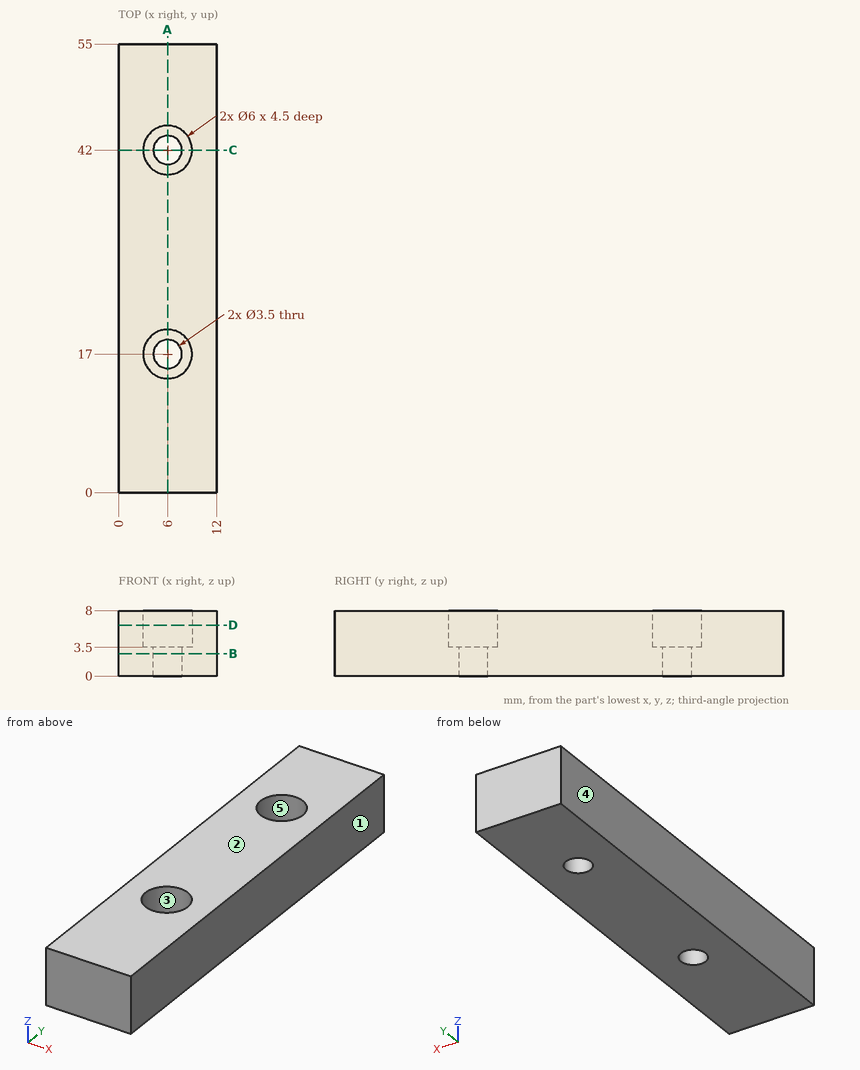
The figure shows three views and two pictorial views of one solid part (mm, origin at its lowest corner). Answer the questions. A direction names the side the tool comes from. Round coordinates to 2 decimals unless told otherwise and drop trailing zeros. Order: outer loops, then holes, each group sorted by start corner. A loop starts at its lowest first (then second) coordinate and runs counter-clockwise, first axis right, second up.
Q1. A tool of negligible diameter and unlimited length cuts with its end or side. For the marked faces 4 and 5, from which of +Z, -Z, +X, -X, +Y, -Y can it reach the whole face along a straight path? Write none if from no direction.
Solution:
face 4: +Z, -Z, -X, +Y, -Y
face 5: +Z
Q2. Given pin 1 Ø2 at (y, z) = (21, 3) entering from -X; pin 2 Ø5 at (x, y) = (6, 17) entering from +Z, each flat-ended and moving along its own axis, determine where each tip first touches the part or whether it passes through.
Solution:
pin 1: stops at x = 0
pin 2: stops at z = 3.5
Q3. Find the intervals of material crossed by line 1 along Y through (x, z) = (6, 1.25); line 2 along Y through (x, z) = (6, 6.2); line 3 along X through (y, z) = (44.5, 4.25), in increasing order.
Solution:
line 1: y = 0 to 15.25, 18.75 to 40.25, 43.75 to 55
line 2: y = 0 to 14, 20 to 39, 45 to 55
line 3: x = 0 to 4.34, 7.66 to 12
Q4. A cutting plane is placed at D-D, the plane z = 6.25. Determine the outline of the cut face in (x, y), then the cut area to 3 significant figures.
Solution:
outline: (0, 0) - (12, 0) - (12, 55) - (0, 55) - close; hole circle Ø6 at (6, 17); hole circle Ø6 at (6, 42)
area: 603 mm2
Q5. A cutting plane is placed at C-C, the plane y = 42. Determine the outline of the cut face in (x, z).
Solution:
outline: (0, 0) - (4.25, 0) - (4.25, 3.5) - (3, 3.5) - (3, 8) - (0, 8) - close; (7.75, 0) - (12, 0) - (12, 8) - (9, 8) - (9, 3.5) - (7.75, 3.5) - close
Q6. A cutting plane is placed at B-B, the plane z = 2.75. Determine the outline of the cut face in (x, y).
Solution:
outline: (0, 0) - (12, 0) - (12, 55) - (0, 55) - close; hole circle Ø3.5 at (6, 17); hole circle Ø3.5 at (6, 42)
Q7. A cutting plane is placed at A-A, the plane x = 6. Determine the outline of the cut face in (y, z).
Solution:
outline: (0, 0) - (15.25, 0) - (15.25, 3.5) - (14, 3.5) - (14, 8) - (0, 8) - close; (18.75, 0) - (40.25, 0) - (40.25, 3.5) - (39, 3.5) - (39, 8) - (20, 8) - (20, 3.5) - (18.75, 3.5) - close; (43.75, 0) - (55, 0) - (55, 8) - (45, 8) - (45, 3.5) - (43.75, 3.5) - close
Q8. The mould has two halves that part along X. Classify the marked faces 1, 2 and 3: pulls with the +X half, pulls with the -X half, needs draft (parallel to the pull), parting line crosses it, or undercut.
Solution:
face 1: pulls with the +X half
face 2: needs draft
face 3: undercut
